from build123d import *

# Parameters (mm, degrees)
F1_DEPTH = 4.064


with BuildPart() as f1:
    # F0 (on Front) → F1 (new body)
    with BuildSketch(Plane.XZ):
        with BuildLine():
            Line((14.949479, 3.175), (0, 3.175))
            Line((0, 3.175), (-14.949479, 3.175))
            ThreePointArc((-14.949479, 3.175), (-22.139438, 4.213873), (-28.741251, 7.245513))
            ThreePointArc((-28.741251, 7.245513), (-32.438266, 8.943231), (-36.464644, 9.525))
            Line((-36.464644, 9.525), (-57.15, 9.525))
            Line((-57.15, 9.525), (-57.15, 0))
            Line((-57.15, 0), (-57.15, -9.525))
            Line((-57.15, -9.525), (-36.464644, -9.525))
            ThreePointArc((-36.464644, -9.525), (-32.438266, -8.943231), (-28.741251, -7.245513))
            ThreePointArc((-28.741251, -7.245513), (-22.139438, -4.213873), (-14.949479, -3.175))
            Line((-14.949479, -3.175), (0, -3.175))
            Line((0, -3.175), (14.949479, -3.175))
            ThreePointArc((14.949479, -3.175), (22.139438, -4.213873), (28.741251, -7.245513))
            ThreePointArc((28.741251, -7.245513), (32.438266, -8.943231), (36.464644, -9.525))
            Line((36.464644, -9.525), (57.15, -9.525))
            Line((57.15, -9.525), (57.15, 0))
            Line((57.15, 0), (57.15, 9.525))
            Line((57.15, 9.525), (36.464644, 9.525))
            ThreePointArc((36.464644, 9.525), (32.438266, 8.943231), (28.741251, 7.245513))
            ThreePointArc((28.741251, 7.245513), (22.139438, 4.213873), (14.949479, 3.175))
        make_face()
    extrude(amount=F1_DEPTH)


solid = f1.part
Input: part model. Units: mm. Frame: model coordinates. A direction names the side the tool comes from. Coordinates: 2 decimals unless noted, no trailing zeros. Order: outer loops, then holes, each group sorted by start corner. A loop starts at its lowest first (then second) coordinate and runs counter-clockwise, first axis right, second up.
1. Cut plane D-D, the plane x = -33.5. Return loops of the section in (y, z).
Checked values:
outline: (-4.06, -9.21) - (0, -9.21) - (0, 9.21) - (-4.06, 9.21) - close
2. Contact query for flat-ended pins moving along their axis: P1, Ø3, axis at x = 4, z = -5.5, coming from the -Y side; P2, Ø1.2, axis at x = -5, y = -2.5, coming from the +Z side (3 decimals). Output: stop coordinate, or through.
Checked values:
P1: passes through
P2: stops at z = 3.175
3. Cut plane A-A, the plane y = -1.25. Return loops of the section in (x, z) (3 decimals).
Checked values:
outline: (-57.15, -9.525) - (-36.465, -9.525) arc R14.224 ccw to (-28.741, -7.246) arc R25.4 cw to (-14.949, -3.175) - (14.949, -3.175) arc R25.4 cw to (28.741, -7.246) arc R14.224 ccw to (36.465, -9.525) - (57.15, -9.525) - (57.15, 9.525) - (36.465, 9.525) arc R14.224 ccw to (28.741, 7.246) arc R25.4 cw to (14.949, 3.175) - (-14.949, 3.175) arc R25.4 cw to (-28.741, 7.246) arc R14.224 ccw to (-36.465, 9.525) - (-57.15, 9.525) - close
4. Draft query along X for faces 4 (the flat face through (57.15, -2, 0)), 5 (the cylindrical face through (-22.237, -2.004, -4.243)), 6 (the flat face through (47, -2, 9.525)). Return one class per face: +X half, -X half, draft (parallel to the pull), parting line (faces both ways), or undercut.
Checked values:
face 4: +X half
face 5: undercut
face 6: draft
5. Cut plane B-B, the plane z = 4.5. Return loops of the section in (x, y).
Checked values:
outline: (-57.15, -4.06) - (-23.05, -4.06) - (-23.05, 0) - (-57.15, 0) - close; (23.05, -4.06) - (57.15, -4.06) - (57.15, 0) - (23.05, 0) - close
6. Cut plane C-C, the plane x = 14. Return loops of the section in (y, z) (3 decimals).
Checked values:
outline: (-4.064, -3.175) - (0, -3.175) - (0, 3.175) - (-4.064, 3.175) - close
7. Access query for faces 1 (the cylindrical face through (32.383, -2.004, -8.927)), 2 (the flat face through (47, -2, -9.525)), 3 (the cylindrical face through (22.237, -2.004, 4.243)). Directions: +Z, -Z, +X, -X, +Y, -Y. A direction counts if a zero-diameter tool reaches every point of the face in a straight line with its end or side. Return the directions, or none.
Checked values:
face 1: -Z, +Y, -Y
face 2: -Z, +X, -X, +Y, -Y
face 3: +Z, +Y, -Y
8. Ray query, line 1 along Z through (x, y) = (-3.5, -2.05) (3 decimals); line 2 along X through (y, z) = (-0.4, -7); line 3 along X through (y, z) = (-0.5, -7.5). Return the intervals inside material, ascending.
Checked values:
line 1: z = -3.175 to 3.175
line 2: x = -57.15 to -28.35, 28.35 to 57.15
line 3: x = -57.15 to -29.15, 29.15 to 57.15
